from build123d import *

# Parameters (mm, degrees)
F0_R      = 8.5
F1_DEPTH  = 18
F1_TAPER  = 9
F2_R      = 4
F3_DEPTH  = 6.1
F5_DEPTH  = 10.6
F6_R      = 2.2
F7_DEPTH  = 9.4
F11_COUNT = 32


with BuildPart() as f1:
    # F0 (on Front) → F1 (new body)
    with BuildSketch(Plane.XZ):
        Circle(F0_R)
    extrude(amount=F1_DEPTH, taper=F1_TAPER)

    # F2 (on face) → F3 (join)
    with BuildSketch(Plane(origin=(0, 0, 0), x_dir=(-1, 0, 0), z_dir=(0, 1, 0))):
        Circle(F2_R)
    extrude(amount=F3_DEPTH)

    # F4 (on face) → F5 (join)
    with BuildSketch(Plane(origin=(0, 6.1, 0), x_dir=(-1, 0, 0), z_dir=(0, 1, 0))):
        Polygon((-0.0899552099, 2.868589908), (-2.5292493383, 1.356391457), (-2.4392941284, -1.512198451), (0.0899552099, -2.868589908), (2.5292493383, -1.356391457), (2.4392941284, 1.512198451), align=None)
    extrude(amount=F5_DEPTH)

    # F6 (on face) → F7 (join)
    with BuildSketch(Plane(origin=(0, 16.7, 0), x_dir=(-1, 0, 0), z_dir=(0, 1, 0))):
        Circle(F6_R)
    extrude(amount=F7_DEPTH)



with BuildPart() as f10:
    # F9 (on face) → F10 section 0
    with BuildSketch(Plane.XZ.offset(18)):
        with BuildLine():
            Line((0.555, 5.6217506779), (0, 6.9361673668))
            Line((0, 6.9361673668), (-0.555, 5.6217506779))
            ThreePointArc((-0.555, 5.6217506779), (0, 5.6490800742), (0.555, 5.6217506779))
        make_face()
    # F8 (on Front) → F10 section 1
    with BuildSketch(Plane.XZ):
        Polygon((0.835, 8.4588873382), (0, 9.3067523038), (-0.835, 8.4588873382), align=None)
    loft()


with BuildPart() as f1_1:
    add(f1.part)

    add(f10.part)  # F11 merges F10
    # F11: F10 ×32 about axis
    f11_axis = Axis((0, -18, 0), (0, 1, 0))
    for i in range(1, F11_COUNT):
        add(f10.part.rotate(f11_axis, i * 360 / F11_COUNT))


solid = f1_1.part
Design review of the part built by this model. Coordinates are the model's own, in mm. A direction names the side the tool comes from. Round coordinates to 2 decimals unless told otherwise and drop trailing zeros. Order: outer loops, then holes, each group sorted by start corner. A loop starts at its lowest first (then second) coordinate and runs counter-clockwise, first axis right, second up. Notation, with made-up numbers: M 79.25,82.25 L 102.25,82.25 A15 ccw 102.25,105.25 Z; hole C 6,32.5 d7. An arc over 180 degrees is marked long. Answer as CSV lines item,"result". Start each with the question number.
1) Wall thickness on line 1 along Z through (x, y) = (-5.75, -14.5); line 2 along Y through (x, z) = (-3.5, 3.5); line 3 along Y through (x, z) = (-0.75, 2.75): over which ranges is each line inside the solid? List them lowest first. Write a range as [from, to].
2) Tool access review of faces 1 (the face through (-1.19, 11.33, 2.18)), 2 (the face through (1.19, 11.33, -2.18)), 3 (the face through (1.293, 11.326, 2.123)), 4 (the face through (-2.1, 21.33, 0.66)), 5 (the face through (-1.293, 11.326, -2.123)): name each direction out of +Z, -Z, +X, -X, +Y, -Y from which nothing blocks a thin tool from reaching the whole face with its end or side.
3) Add section B-B (y = 3). Give the boundary of the cut face in (x, z), then the cut area to 3 significant figures.
4) For pin 1 Ø6 at (x, y) = (4.5, -7.5) entering from +Z; pin 2 Ø3 at (y, z) = (16.5, -3.5) entering from -X; pin 3 Ø4 at (x, y) = (2.5, 9) entering from -Z, all flat-tipped, find the tip position at first contact; note any pin that passes through.
5) Add section C-C (y = 18.5). Give the boundary of the cut face in (x, z), then the cut area to 3 significant figures.
6) Add section A-A (y = 12). Give the boundary of the cut face in (x, z).
Resolved:
1,line 1,"[-4.06, -3.41], [-2.91, 2.91], [3.41, 4.06]"
1,line 2,"[-18, 0]"
1,line 3,"[-18, 6.1]"
2,face 1,"+Z, -X, +Y"
2,face 2,"-Z, +X, +Y"
2,face 3,"+Z, +X, +Y"
2,face 4,"+Y"
2,face 5,"-Z, -X, +Y"
3,outline,"C 0,0 d8"
3,area,"50.3 mm^2"
4,pin 1,"z = 8.28"
4,pin 2,"x = -1.49"
4,pin 3,"z = -2.55"
5,outline,"C 0,0 d4.4"
5,area,"15.2 mm^2"
6,outline,"M -2.53,-1.36 L -0.09,-2.87 L 2.44,-1.51 L 2.53,1.36 L 0.09,2.87 L -2.44,1.51 Z"
